from build123d import *

# Parameters (mm, degrees)
SKETCH1_W           = 44.45
SKETCH1_H           = 88.9
SKETCH1_R           = 7.9375
SKETCH1_R_2         = 17.4625
BOSS_EXTRUDE1_DEPTH = 50.8
SKETCH5_R           = 2.032
CUT_EXTRUDE1_DEPTH  = 112.622813528
SKETCH5_3_R         = 3.5
CUT_EXTRUDE2_DEPTH  = 15.1765
CUT_EXTRUDE3_DEPTH  = 2.54
FILLET1_R           = 1.27


with BuildPart() as part:
    # Sketch1 → Boss-Extrude1 (new body)
    with BuildSketch(Plane(origin=(0, 0, 0), x_dir=(0, 0, -1), z_dir=(1, 0, 0))):
        with Locations((22.225, 44.45)):
            Rectangle(SKETCH1_W, SKETCH1_H)
        with Locations(Location((22.225, 19.685, 0), (0, 0, 180))):
            Circle(SKETCH1_R, mode=Mode.SUBTRACT)
        with Locations(Location((22.225, 60.325, 0), (0, 0, 180))):
            Circle(SKETCH1_R_2, mode=Mode.SUBTRACT)
    extrude(amount=BOSS_EXTRUDE1_DEPTH)

    # Sketch5 → Cut-Extrude1 (cut, through all)
    with BuildSketch(Plane.XY):
        with Locations((12.7, 83.34375)):
            Circle(SKETCH5_R)
        with Locations((12.7, 35.2425)):
            Circle(SKETCH5_R)
        with Locations((38.1, 83.34375)):
            Circle(SKETCH5_R)
        with Locations((38.1, 35.2425)):
            Circle(SKETCH5_R)
        with Locations((12.7, 5.87375)):
            Circle(SKETCH5_R)
        with Locations((38.1, 5.87375)):
            Circle(SKETCH5_R)
    extrude(amount=-CUT_EXTRUDE1_DEPTH, mode=Mode.SUBTRACT)

    # Sketch5<3> → Cut-Extrude2 (cut)
    with BuildSketch(Plane.XY):
        with Locations((38.1, 35.2425)):
            Circle(SKETCH5_3_R)
        with Locations((12.7, 83.34375)):
            Circle(SKETCH5_3_R)
        with Locations((38.1, 83.34375)):
            Circle(SKETCH5_3_R)
        with Locations((12.7, 35.2425)):
            Circle(SKETCH5_3_R)
        with Locations((38.1, 5.87375)):
            Circle(SKETCH5_3_R)
        with Locations((12.7, 5.87375)):
            Circle(SKETCH5_3_R)
    extrude(amount=-CUT_EXTRUDE2_DEPTH, mode=Mode.SUBTRACT)

    # Sketch6 → Cut-Extrude3 (cut)
    with BuildSketch(Plane(origin=(0, 0, -44.45), x_dir=(-1, 0, 0), z_dir=(0, 0, -1))):
        Polygon((-8.636, 83.34375), (-10.668, 86.863277241), (-14.732, 86.863277241), (-16.764, 83.34375), (-14.732, 79.824222759), (-10.668, 79.824222759), align=None)
        Polygon((-34.036, 83.34375), (-36.068, 86.863277241), (-40.132, 86.863277241), (-42.164, 83.34375), (-40.132, 79.824222759), (-36.068, 79.824222759), align=None)
        Polygon((-34.036, 35.2425), (-36.068, 38.762027241), (-40.132, 38.762027241), (-42.164, 35.2425), (-40.132, 31.722972759), (-36.068, 31.722972759), align=None)
        Polygon((-8.636, 35.2425), (-10.668, 38.762027241), (-14.732, 38.762027241), (-16.764, 35.2425), (-14.732, 31.722972759), (-10.668, 31.722972759), align=None)
        Polygon((-8.636, 5.87375), (-10.668, 9.393277241), (-14.732, 9.393277241), (-16.764, 5.87375), (-14.732, 2.354222759), (-10.668, 2.354222759), align=None)
        Polygon((-34.036, 5.87375), (-36.068, 9.393277241), (-40.132, 9.393277241), (-42.164, 5.87375), (-40.132, 2.354222759), (-36.068, 2.354222759), align=None)
    extrude(amount=-CUT_EXTRUDE3_DEPTH, mode=Mode.SUBTRACT)

    # Fillet1
    fillet1_edges = [part.edges().sort_by_distance(p)[0] for p in [
        (0, 60.325, -39.6875),
        (50.8, 60.325, -39.6875),
        (50.8, 88.9, -22.225),
        (0, 19.685, -30.1625),
        (50.8, 19.685, -30.1625),
        (50.8, 44.45, 0),
        (50.8, 0, -22.225),
        (0, 44.45, 0),
        (0, 88.9, -22.225),
        (0, 44.45, -44.45),
        (0, 0, -22.225),
        (25.4, 0, 0),
        (25.4, 88.9, 0),
        (25.4, 88.9, -44.45),
        (25.4, 0, -44.45),
        (50.8, 44.45, -44.45),
    ]]
    fillet(fillet1_edges, radius=FILLET1_R)

    # SurfaceCut1
    split(bisect_by=Plane.XY.offset(-22.225), keep=Keep.TOP)


solid = part.part
Geometry check sheet. Reference: the model listing, model coordinates, mm. A direction names the side the tool comes from. Coordinates: 2 decimals unless noted, no trailing zeros. Use a Markdown table: item, result. Add a question column.
1. Material ranges on L1, parallel to X at y = 6, z = -4.25; L2, parallel to Y at x = 12.7, z = -8.5; L3, parallel to Y at x = 12.5, z = -19.5, recorded low to high.
2. Mould release check, pull along Y, two halves, no side actions. Record for faces 1 (the face through (25, 0, -12)), 2 (the face through (25, 83, -22.225)), 3 (the face through (16.038, 6.925, -7.482)): pulls with the +Y half, pulls with the -Y half, needs draft (parallel to the pull), parting line crosses it, or undercut.
3. Cross-section at A-A (x = 12.7). Give the number of separate pieces and of enclosed holes in the cut face, and give its area (3 significant figures).
4. Set-up check for faces 4 (the face through (25.062, 60.709, -4.767)), 5 (the face through (39.72, 80.24, -7.48)): record each of +Z, -Z, +X, -X, +Y, -Y from which the full face is reachable in a straight line by a thin tool's end or side.
5. Go/stop test with flat-tipped pins: pin 1 Ø1 at (x, y) = (28, 45) entering from +Z; pin 2 Ø2 at (x, y) = (37.5, 37) entering from +Z; pin 3 Ø3.5 at (x, y) = (38.1, 5.87) entering from -Z. Record where each tip stops, or that it passes through.
Filled sheet:
| question | item | result |
|---|---|---|
| 1 | L1 | 0 to 9.2, 16.2 to 34.6, 41.6 to 50.8 |
| 1 | L2 | 0 to 2.37, 9.37 to 31.74, 38.74 to 49.53, 71.12 to 79.84, 86.84 to 88.9 |
| 1 | L3 | 0 to 3.85, 7.9 to 12.23, 27.14 to 33.22, 37.26 to 43.08, 77.57 to 81.32, 85.37 to 88.9 |
| 2 | face 1 | pulls with the -Y half |
| 2 | face 2 | needs draft |
| 2 | face 3 | undercut |
| 3 | separate pieces | 4 |
| 3 | enclosed holes | 0 |
| 3 | area | 993 mm2 |
| 4 | face 4 | -Z, +X, -X |
| 4 | face 5 | +Z |
| 5 | pin 1 | z = 0 |
| 5 | pin 2 | z = -15.18 |
| 5 | pin 3 | through |
